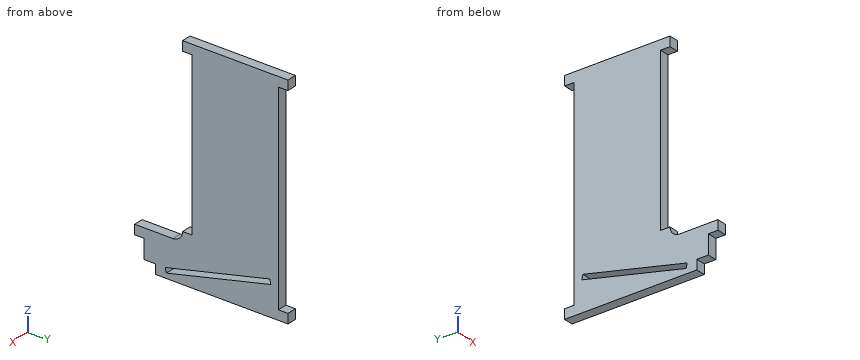
```python
from build123d import *

# Parameters (mm, degrees)
F0_W      = 31.75
F0_H      = 25.4
F1_DEPTH  = 6.35
F2_W      = 6.35
F2_H      = 133.35
F3_DEPTH  = 12.446
F4_W      = 6.35
F4_H      = 107.95
F5_DEPTH  = 9.906
F6_W      = 7.62
F6_H      = 6.35
F7_DEPTH  = 10.668
F8_W      = 6.35
F8_H      = 6.35
F9_DEPTH  = 6.35
F10_R     = 6.35
F11_DEPTH = 8.9408
F13_DEPTH = 6.351


with BuildPart() as f1:
    # F0 (on Right) → F1 (new body)
    with BuildSketch(Plane.YZ):
        Polygon((-69.85, 0), (0, 0), (0, 146.05), (-69.85, 146.05), (-69.85, 25.4), align=None)
        with Locations((-85.725, 12.7)):
            Rectangle(F0_W, F0_H)
    extrude(amount=F1_DEPTH)

    # F2 (on Right) → F3 (cut)
    with BuildSketch(Plane.YZ):
        with Locations((-3.175, 73.025)):
            Rectangle(F2_W, F2_H)
    extrude(amount=F3_DEPTH, mode=Mode.SUBTRACT)

    # F4 (on Right) → F5 (cut)
    with BuildSketch(Plane.YZ):
        with Locations((-66.675, 85.725)):
            Rectangle(F4_W, F4_H)
    extrude(amount=F5_DEPTH, mode=Mode.SUBTRACT)

    # F6 (on Right) → F7 (cut)
    with BuildSketch(Plane.YZ):
        Polygon((-95.25, 19.05), (-101.6, 19.05), (-101.6, 0), (-95.25, 0), (-95.25, 6.35), align=None)
        with Locations((-91.44, 3.175)):
            Rectangle(F6_W, F6_H)
    extrude(amount=F7_DEPTH, mode=Mode.SUBTRACT)

    # F8 (on Right) → F9 (join)
    with BuildSketch(Plane.YZ):
        with Locations((-73.025, 28.575)):
            Rectangle(F8_W, F8_H)
    extrude(amount=F9_DEPTH)

    # F10 (on Right) → F11 (cut)
    with BuildSketch(Plane.YZ):
        with Locations((-76.2, 31.75)):
            Circle(F10_R)
    extrude(amount=F11_DEPTH, mode=Mode.SUBTRACT)

    # F12 (on face) → F13 (cut, through all)
    with BuildSketch(Plane(origin=(0, 0, 0), x_dir=(0, -1, 0), z_dir=(-1, 0, 0))):
        Polygon((80.54212, 3.261933), (81.28, 6.35), (12.107297, 22.878509), (11.369418, 19.790442), align=None)
    extrude(amount=-F13_DEPTH, mode=Mode.SUBTRACT)


solid = f1.part
```
Design review of the part built by this model. Coordinates are the model's own, in mm. Coordinates: 2 decimals unless noted, no trailing zeros. Order: outer loops, then holes, each group sorted by start corner. A loop starts at its lowest first (then second) coordinate and runs counter-clockwise, first axis right, second up. Notation, with made-up numbers: (41, 67) - (73, 67) arc R22 ccw to (73, 80) - close; hole circle Ø2 at (68, 26). An arc over 180 degrees is marked (long way). One line per question, with ' | ' between items.
Q1. Consider section A-A, the plane x = 2.5. Give the boundary of the cut face in (y, z), then the cut area to 3 significant figures.
Answer key:
outline: (-101.6, 19.05) - (-95.25, 19.05) - (-95.25, 6.35) - (-87.63, 6.35) - (-87.63, 0) - (0, 0) - (0, 6.35) - (-6.35, 6.35) - (-6.35, 139.7) - (0, 139.7) - (0, 146.05) - (-69.85, 146.05) - (-69.85, 139.7) - (-63.5, 139.7) - (-63.5, 31.75) - (-69.85, 31.75) arc R6.35 cw to (-76.2, 25.4) - (-101.6, 25.4) - close; hole (-81.28, 6.35) - (-80.54, 3.26) - (-11.37, 19.79) - (-12.11, 22.88) - close | area: 9,090 mm2
Q2. To check wall thickness, follow line 1 along Y through (x, z) = (0.5, 134.5); line 2 along Z through (x, y) = (6.25, -47); line 3 along Z through (x, y) = (6.25, -87). State the ranges of each line that lie inside material, in increasing order.
Answer key:
line 1: y = -63.5 to -6.35 | line 2: z = 0 to 11.28, 14.54 to 146.05 | line 3: z = 0 to 25.4
Q3. Consider section C-C, the plane z = 38.5. Give the boundary of the cut face in (x, y), then the cut area to 3 significant figures.
Answer key:
outline: (0, -63.5) - (6.35, -63.5) - (6.35, -6.35) - (0, -6.35) - close | area: 363 mm2
Q4. Clearance check with flat-ended pins moving along their axes: pin 1 Ø3 at (x, z) = (4, 2.5) entering from -Y; pin 2 Ø3 at (x, z) = (5, 78) entering from +Y; pin 3 Ø3 at (x, y) = (4, -2.5) entering from -Z; pin 4 Ø1.9 at (x, z) = (3, 143.5) entering from -Y. State where each tip first meets the part, or that it passes through.
Answer key:
pin 1: stops at y = -87.63 | pin 2: stops at y = -6.35 | pin 3: stops at z = 0 | pin 4: stops at y = -69.85
Q5. Consider section B-B, the plane y = -62. Give the boundary of the cut face in (x, z).
Answer key:
outline: (0, 0) - (6.35, 0) - (6.35, 7.69) - (0, 7.69) - close; (0, 10.96) - (6.35, 10.96) - (6.35, 146.05) - (0, 146.05) - close
